```python
from build123d import *

# Parameters (mm, degrees)
SKETCH_1_W          = 86
SKETCH_1_H          = 44.4
EXTRUDE_1_DEPTH     = 19.6
EXTRUDE_2_DEPTH     = 5
SKETCH_3_W          = 83.2
SKETCH_3_H          = 42
CUT_EXTRUDE_1_DEPTH = 18.4
FILLET_1_R          = 3


with BuildPart() as part:
    # Эскиз1 → Бобышка-Вытянуть1 (new body)
    with BuildSketch(Plane.XY):
        Rectangle(SKETCH_1_W, SKETCH_1_H)
    extrude(amount=EXTRUDE_1_DEPTH)

    # Эскиз2 → Бобышка-Вытянуть2 (add)
    with BuildSketch(Plane.XY):
        with BuildLine():
            Line((43, 17.2), (43, 13.108775687))
            ThreePointArc((43, 13.108775687), (53.273546839, 0), (43, -13.108775687))
            Line((43, -13.108775687), (43, -17.2))
            ThreePointArc((43, -17.2), (57.273546839, 0), (43, 17.2))
        make_face()
    extrude(amount=EXTRUDE_2_DEPTH)

    # Эскиз3 → Вырез-Вытянуть1 (cut)
    with BuildSketch(Plane.XY.offset(19.6)):
        with Locations((0.2, 0)):
            Rectangle(SKETCH_3_W, SKETCH_3_H)
    extrude(amount=-CUT_EXTRUDE_1_DEPTH, mode=Mode.SUBTRACT)

    # Скругление1
    fillet_1_edges = [part.edges().sort_by_distance(p)[0] for p in [
        (-41.4, -21, 10.4),
        (-41.4, 21, 10.4),
        (-43, -22.2, 9.8),
        (-43, 22.2, 9.8),
    ]]
    fillet(fillet_1_edges, radius=FILLET_1_R)


solid = part.part
```
The model under review builds one solid part; all positions refer to its coordinate system, in mm. A direction names the side the tool comes from. Give positions to 0.01 mm unless a question says otherwise; leave off trailing zeros. Write each loop counter-clockwise with the first axis right and the second up, starting at its lowest first coordinate (ties: lowest second). Pieces come first, ordered by that corner, then holes.
(1) The part is to be moulded in two halves that separate along X. For faces 1 (the cylindrical face through (57.27, -0.34, 2.46)), 2 (the flat face through (-41.4, 0, 11)), 3 (the flat face through (6, 0, 0)), say which applies: released by +X, released by -X, zero draft, split by the parting line, or undercut.
(2) For P1, Ø8, axis at x = -13.5, y = 15.5, coming from the +Z side; P2, Ø8, axis at y = 17, z = 13.5, coming from the +X side; P3, Ø7, axis at x = 53, y = -4, coming from the +Z side, all flat-tipped, find the tip position at first contact; note any pin that passes through.
(3) Tool access review of faces 4 (the flat face through (53.3, -2.5, 5)), 5 (the flat face through (43, 0, 10)), 6 (the cylindrical face through (-42.14, -21.3, 9.94)): name each direction out of +Z, -Z, +X, -X, +Y, -Y from which nothing blocks a thin tool from reaching the whole face with its end or side.
(4) Consider section B-B, the plane x = -12. Give the boundary of the cut face in (y, z).
(5) Consider section C-C, the plane y = -5. Give the boundary of the cut face in (x, z).
(6) To check wall thickness, follow L1, parallel to Y at x = 26.5, z = 12; L2, parallel to X at y = -5.5, z = 18.25; L3, parallel to X at y = -0.5, z = 1. State the ranges of each line that lie inside material, in increasing order.
(7) Consider section A-A, the plane z = 17. Give the boundary of the cut face in (x, y).
(8) Consider section D-D, the plane y = 16. Give the boundary of the cut face in (x, z).
Returned:
1. face 1: released by +X
1. face 2: undercut
1. face 3: zero draft
2. P1: stops at z = 1.2
2. P2: stops at x = 43
2. P3: stops at z = 5
3. face 4: +Z, +X, +Y, -Y
3. face 5: +Z
3. face 6: +Z, -Z, -X, -Y
4. outline: (-22.2, 0) - (22.2, 0) - (22.2, 19.6) - (21, 19.6) - (21, 1.2) - (-21, 1.2) - (-21, 19.6) - (-22.2, 19.6) - close
5. outline: (-43, 0) - (43, 0) - (43, 19.6) - (41.8, 19.6) - (41.8, 1.2) - (-41.4, 1.2) - (-41.4, 19.6) - (-43, 19.6) - close; (52.31, 0) - (56.54, 0) - (56.54, 5) - (52.31, 5) - close
6. L1: y = -22.2 to -21, 21 to 22.2
6. L2: x = -43 to -41.4, 41.8 to 43
6. L3: x = -43 to 43, 53.26 to 57.27
7. outline: (-43, -19.2) arc R3 ccw to (-40, -22.2) - (43, -22.2) - (43, 22.2) - (-40, 22.2) arc R3 ccw to (-43, 19.2) - close; hole (-41.4, -18) arc R3 ccw to (-38.4, -21) - (41.8, -21) - (41.8, 21) - (-38.4, 21) arc R3 ccw to (-41.4, 18) - close
8. outline: (-43, 0) - (46.86, 0) - (46.86, 5) - (43, 5) - (43, 19.6) - (41.8, 19.6) - (41.8, 1.2) - (-41.4, 1.2) - (-41.4, 19.6) - (-43, 19.6) - close
